Could you check a few things on this model? Use its own coordinates, in mm. A direction names the side the tool comes from. Give positions to 0.01 mm unless a question says otherwise; leave off trailing zeros. Write each loop counter-clockwise with the first axis right and the second up, starting at its lowest first coordinate (ties: lowest second). Pieces come first, ordered by that corner, then holes. Notation, with made-up numbers: (49.25, 49.25) -> (86.25, 49.25) arc R29 cw to (86.25, 80.25) -> close; hole circle Ø3 at (54, 32.25). An arc over 180 degrees is marked (long way). One line per question, with ' | ' between items.
from build123d import *

# Parameters (mm, degrees)
BOSS_EXTRUDE1_DEPTH      = 2
BOSS_EXTRUDE1_DEPTH_BACK = 3
BOSS_EXTRUDE2_START      = -2
SKETCH2_W                = 22.4
SKETCH2_H                = 3
BOSS_EXTRUDE2_DEPTH      = 2


with BuildPart() as part:
    # Sketch1 → Boss-Extrude1 (new, two sides: drawn at the far end of the back side and taken through both)
    with BuildSketch(Plane.XY.offset(-BOSS_EXTRUDE1_DEPTH_BACK)):
        with BuildLine():
            Line((-34.384444189, 19.919216619), (-7.984444189, 19.919216619))
            ThreePointArc((-7.984444189, 19.919216619), (8.465555811, 3.469216619), (-7.984444189, -12.980783381))
            Line((-7.984444189, -12.980783381), (-34.384444189, -12.980783381))
            ThreePointArc((-34.384444189, -12.980783381), (-50.834444189, 3.469216619), (-34.384444189, 19.919216619))
        make_face()
        with BuildLine():
            Line((-34.384444189, 18.719216619), (-7.984444189, 18.719216619))
            ThreePointArc((-7.984444189, 18.719216619), (7.265555811, 3.469216619), (-7.984444189, -11.780783381))
            Line((-7.984444189, -11.780783381), (-34.384444189, -11.780783381))
            ThreePointArc((-34.384444189, -11.780783381), (-49.634444189, 3.469216619), (-34.384444189, 18.719216619))
        make_face(mode=Mode.SUBTRACT)
    extrude(amount=BOSS_EXTRUDE1_DEPTH + BOSS_EXTRUDE1_DEPTH_BACK)

    # Sketch2 → Boss-Extrude2 (add)
    with BuildSketch(Plane.XY.offset(2).offset(BOSS_EXTRUDE2_START)):
        with BuildLine():
            ThreePointArc((-5.984444189, -11.649067014), (7.265555811, 3.469216619), (-5.984444189, 18.587500252))
            Line((-5.984444189, 18.587500252), (-5.984444189, 15.554848584))
            ThreePointArc((-5.984444189, 15.554848584), (4.265555811, 3.469216619), (-5.984444189, -8.616415346))
            Line((-5.984444189, -8.616415346), (-5.984444189, -11.649067014))
        make_face()
        with Locations((-21.184444189, 17.219216619)):
            Rectangle(SKETCH2_W, SKETCH2_H)
        with Locations((-21.184444189, -10.280783381)):
            Rectangle(SKETCH2_W, SKETCH2_H)
        with BuildLine():
            ThreePointArc((-36.384444189, -8.616415346), (-46.634444189, 3.469216619), (-36.384444189, 15.554848584))
            Line((-36.384444189, 15.554848584), (-36.384444189, 18.587500252))
            ThreePointArc((-36.384444189, 18.587500252), (-49.634444189, 3.469216619), (-36.384444189, -11.649067014))
            Line((-36.384444189, -11.649067014), (-36.384444189, -8.616415346))
        make_face()
    extrude(amount=BOSS_EXTRUDE2_DEPTH)


solid = part.part
Q1. If I drill on line 1 along Y through (x, z) = (-12, 1.55); line 2 along Y through (x, z) = (-15, -1.2); line 3 along Z through (x, y) = (-29, -9.5), over which ranges is the centre line in solid material (lowest first)?
Answer below:
line 1: y = -12.98 to -8.78, 15.72 to 19.92 | line 2: y = -12.98 to -11.78, 18.72 to 19.92 | line 3: z = 0 to 2
Q2. On a 3-axis mill with a long thin cutter (end or side, diameter ignored), from which of +Z, -Z, +X, -X, +Y, -Y can I reach the whole of each face in a straight line? I mean faces 4 (the flat face through (-5.984, 17, 1)), 5 (the cylindrical face through (8.46, 3.83, -0.54)), 6 (the cylindrical face through (7.26, 3.8, -1.65)). Say none if no direction works.
Answer below:
face 4: +Z, -Z | face 5: +Z, -Z, +X | face 6: -Z
Q3. Will these pins go through, and if not, where does the flat tip stop? pin 1 (1.5 mm diameter, centred on y = -0.5, z = -0.5, fed in from -X); pin 2 (2 mm diameter, centred on y = -10, z = 1, fed in from +X) (3 decimals); pin 3 (5 mm diameter, centred on x = -43, y = 12.5, fed in from -Z); pin 4 (3 mm diameter, centred on x = -14.5, y = 15, fed in from +Z).
Answer below:
pin 1: stops at x = -50.52 | pin 2: stops at x = 2.745 | pin 3: stops at z = 0 | pin 4: stops at z = 2
Q4. Imagine slicing it at B-B on x = -31. Please give me the cut outline in (y, z).
Answer below:
outline: (-12.98, -3) -> (-11.78, -3) -> (-11.78, 0) -> (-8.78, 0) -> (-8.78, 2) -> (-12.98, 2) -> close; (15.72, 0) -> (18.72, 0) -> (18.72, -3) -> (19.92, -3) -> (19.92, 2) -> (15.72, 2) -> close
Q5. Imagine slicing it at A-A on z = -1.95. Please give me the cut outline in (x, y), and give its area (3 significant figures).
Answer below:
outline: (-34.38, -12.98) -> (-7.98, -12.98) arc R16.45 ccw to (-7.98, 19.92) -> (-34.38, 19.92) arc R16.45 ccw to start; hole (-34.38, -11.78) -> (-7.98, -11.78) arc R15.25 ccw to (-7.98, 18.72) -> (-34.38, 18.72) arc R15.25 ccw to start | area: 183 mm^2
Q6. If we mould it in two halves opening along X, with no side actions, what happens to faces 1 (the flat face through (-23, 16, 2)), 2 (the cylindrical face through (-50.83, 3.11, -0.54)), 3 (the flat face through (-21, 17, 0))? For each: +X half, -X half, draft (parallel to the pull), parting line (faces both ways), or undercut.
Answer below:
face 1: draft | face 2: -X half | face 3: undercut
Q7. Imagine slicing it at D-D on y = -11. Please give me the cut outline in (x, z).
Answer below:
outline: (-42.21, -3) -> (-39.2, -3) -> (-39.2, 0) -> (-36.38, 0) -> (-36.38, 2) -> (-42.21, 2) -> close; (-32.38, 0) -> (-9.98, 0) -> (-9.98, 2) -> (-32.38, 2) -> close; (-5.98, 0) -> (-3.17, 0) -> (-3.17, -3) -> (-0.16, -3) -> (-0.16, 2) -> (-5.98, 2) -> close
Q8. Imagine slicing it at C-C on y = 4. Please give me the cut outline in (x, z), and give its area (3 significant figures).
Answer below:
outline: (-50.83, -3) -> (-49.63, -3) -> (-49.63, 0) -> (-46.62, 0) -> (-46.62, 2) -> (-50.83, 2) -> close; (4.25, 0) -> (7.26, 0) -> (7.26, -3) -> (8.46, -3) -> (8.46, 2) -> (4.25, 2) -> close | area: 24.0 mm^2
